Input: part model. Units: mm. Frame: model coordinates. A direction names the side the tool comes from. Round coordinates to 2 decimals unless told otherwise and drop trailing zeros. Loops run counter-clockwise (first coordinate to the right, second up) from the corner with the lowest first, then second, coordinate; pieces in that order, holes last. Notation, with made-up numbers: (88.5, 51.25) -> (95.5, 51.25) arc R18 cw to (95.5, 74.25) -> close; hole circle Ø7 at (30, -34.75). An arc over 180 degrees is marked (long way). Answer as a JSON object with one key per item and string values.
```python
from build123d import *

# Parameters (mm, degrees)
SKETCH1_R                              = 26.25
BOSS_EXTRUDE1_DEPTH                    = 105
BOSS_EXTRUDE2_DEPTH                    = 52.5
TAP_DRILL_FOR_M24X2_0_TAP1_D           = 22
TAP_DRILL_FOR_M24X2_0_TAP1_DEPTH       = 105
TAP_DRILL_FOR_M24X2_0_TAP1_CSINK_D     = 22.05
TAP_DRILL_FOR_M24X2_0_TAP1_CSINK_ANGLE = 90
TAP_DRILL_FOR_M24X2_0_TAP1_TIP         = 6.609466809
BOSS_EXTRUDE3_DEPTH                    = 40
FILLET1_R                              = 5
TAP_DRILL_FOR_M42X3_0_TAP1_D           = 39
TAP_DRILL_FOR_M42X3_0_TAP1_CSINK_D     = 39.05
TAP_DRILL_FOR_M42X3_0_TAP1_CSINK_ANGLE = 90


with BuildPart() as part:
    # Sketch1 → Boss-Extrude1 (new body)
    with BuildSketch(Plane(origin=(0, 0, 0), x_dir=(0, 0, -1), z_dir=(1, 0, 0))):
        Circle(SKETCH1_R)
    extrude(amount=BOSS_EXTRUDE1_DEPTH)

    # Sketch2 → Boss-Extrude2 (add)
    with BuildSketch(Plane(origin=(105, 0, 0), x_dir=(0, 0, -1), z_dir=(1, 0, 0))):
        with BuildLine():
            Line((-26.25, 0), (-26.25, -105))
            Line((-26.25, -105), (26.25, -105))
            Line((26.25, -105), (26.25, 0))
            ThreePointArc((26.25, 0), (0, 26.25), (-26.25, 0))
        make_face()
    extrude(amount=BOSS_EXTRUDE2_DEPTH)

    # Tap Drill for M24x2.0 Tap1
    with Locations(Plane.ZY):
        with Locations((0, 0)):
            CounterSinkHole(TAP_DRILL_FOR_M24X2_0_TAP1_D / 2, TAP_DRILL_FOR_M24X2_0_TAP1_CSINK_D / 2, depth=TAP_DRILL_FOR_M24X2_0_TAP1_DEPTH, counter_sink_angle=TAP_DRILL_FOR_M24X2_0_TAP1_CSINK_ANGLE)
            with Locations((0, 0, -(TAP_DRILL_FOR_M24X2_0_TAP1_DEPTH + TAP_DRILL_FOR_M24X2_0_TAP1_TIP / 2))):  # 118° drill point
                Cone(0, TAP_DRILL_FOR_M24X2_0_TAP1_D / 2, TAP_DRILL_FOR_M24X2_0_TAP1_TIP, mode=Mode.SUBTRACT)

    # Sketch7 → Boss-Extrude3 (add)
    with BuildSketch(Plane.XZ.offset(105)):
        Polygon((52.5, 300), (352.5, 300), (352.5, -300), (52.5, -300), (52.5, 0), align=None)
    extrude(amount=BOSS_EXTRUDE3_DEPTH)

    # Fillet1
    fillet1_edges = [part.edges().sort_by_distance(p)[0] for p in [
        (105, -105, 0),
        (131.25, -105, 26.25),
        (131.25, -105, -26.25),
        (157.5, -105, 0),
    ]]
    fillet(fillet1_edges, radius=FILLET1_R)

    # Tap Drill for M42x3.0 Tap1 (through all)
    with Locations(Plane(origin=(0, -105, 0), x_dir=(1, 0, 0), z_dir=(0, 1, 0))):
        with Locations((302.5, -250), (302.5, 250)):
            CounterSinkHole(TAP_DRILL_FOR_M42X3_0_TAP1_D / 2, TAP_DRILL_FOR_M42X3_0_TAP1_CSINK_D / 2, counter_sink_angle=TAP_DRILL_FOR_M42X3_0_TAP1_CSINK_ANGLE)


solid = part.part
```
1) Contact query for flat-ended pins moving along their axis: P1, Ø6, axis at x = 138.5, y = -46.5, coming from the +Z side; P2, Ø2, axis at y = 1, z = 10, coming from the +X side; P3, Ø20, axis at y = -126, z = 7.5, coming from the -X side. Output: stop coordinate, or through.
Output:
{"P1": "stops at z = 26.25", "P2": "stops at x = 157.5", "P3": "stops at x = 52.5"}
2) Section B-B, the plane x = 302.5. Output: boundary loops of the cut face in (y, z) (3 decimals), plus the area to 3 significant figures.
Output:
{"outline": "(-145, -300) -> (-105, -300) -> (-105, -269.525) -> (-105.025, -269.5) -> (-145, -269.5) -> close; (-145, -230.5) -> (-105.025, -230.5) -> (-105, -230.475) -> (-105, 230.475) -> (-105.025, 230.5) -> (-145, 230.5) -> close; (-145, 269.5) -> (-105.025, 269.5) -> (-105, 269.525) -> (-105, 300) -> (-145, 300) -> close", "area": "20,900 mm^2"}
3) Section A-A, the plane z = 250. Output: boundary loops of the cut face in (x, y) (3 decimals), plus the area to 3 significant figures.
Output:
{"outline": "(52.5, -145) -> (283, -145) -> (283, -105.025) -> (282.975, -105) -> (52.5, -105) -> close; (322, -145) -> (352.5, -145) -> (352.5, -105) -> (322.025, -105) -> (322, -105.025) -> close", "area": "10,400 mm^2"}
4) Draft query along Y for faces 1 (the face through (131, -51, -26.25)), 2 (the face through (60.148, 26.027, 3.417)). Return one class per face: +Y half, -Y half, draft (parallel to the pull), parting line (faces both ways), or undercut.
Output:
{"face 1": "draft", "face 2": "undercut"}
5) Section D-D, the plane y = -40. Output: boundary loops of the cut face in (x, z).
Output:
{"outline": "(105, -26.25) -> (157.5, -26.25) -> (157.5, 26.25) -> (105, 26.25) -> close"}
6) Ray query, probe 1 along Z at (x, y) = (302.5, -124); probe 2 along X at (y, z) = (-120, 250); probe 3 along Y at (x, z) = (81, 5). Return the intervals inside material, ascending.
Output:
{"probe 1": "z = -300 to -269.5, -230.5 to 230.5, 269.5 to 300", "probe 2": "x = 52.5 to 283, 322 to 352.5", "probe 3": "y = -145 to -105, -25.77 to -9.8, 9.8 to 25.77"}
7) Reachability of faces 3 (the face through (352.5, -125, 4)), 4 (the face through (131, -49, 26.25)), 5 (the face through (157.5, -36, 0)), 6 (the face through (53.25, -10.74, 2.38)) from +Z, -Z, +X, -X, +Y, -Y: full face, straight path, thin tool, end or side. Return the list, or none.
Output:
{"face 3": "+Z, -Z, +X, +Y, -Y", "face 4": "+Z, +X, -X, +Y", "face 5": "+Z, -Z, +X, +Y", "face 6": "-X"}
8) Section C-C, the plane x = 149. Output: boundary loops of the cut face in (y, z).
Output:
{"outline": "(-145, -300) -> (-105, -300) -> (-105, -31.25) arc R5 cw to (-100, -26.25) -> (0, -26.25) arc R26.25 ccw to (0, 26.25) -> (-100, 26.25) arc R5 cw to (-105, 31.25) -> (-105, 300) -> (-145, 300) -> close"}
